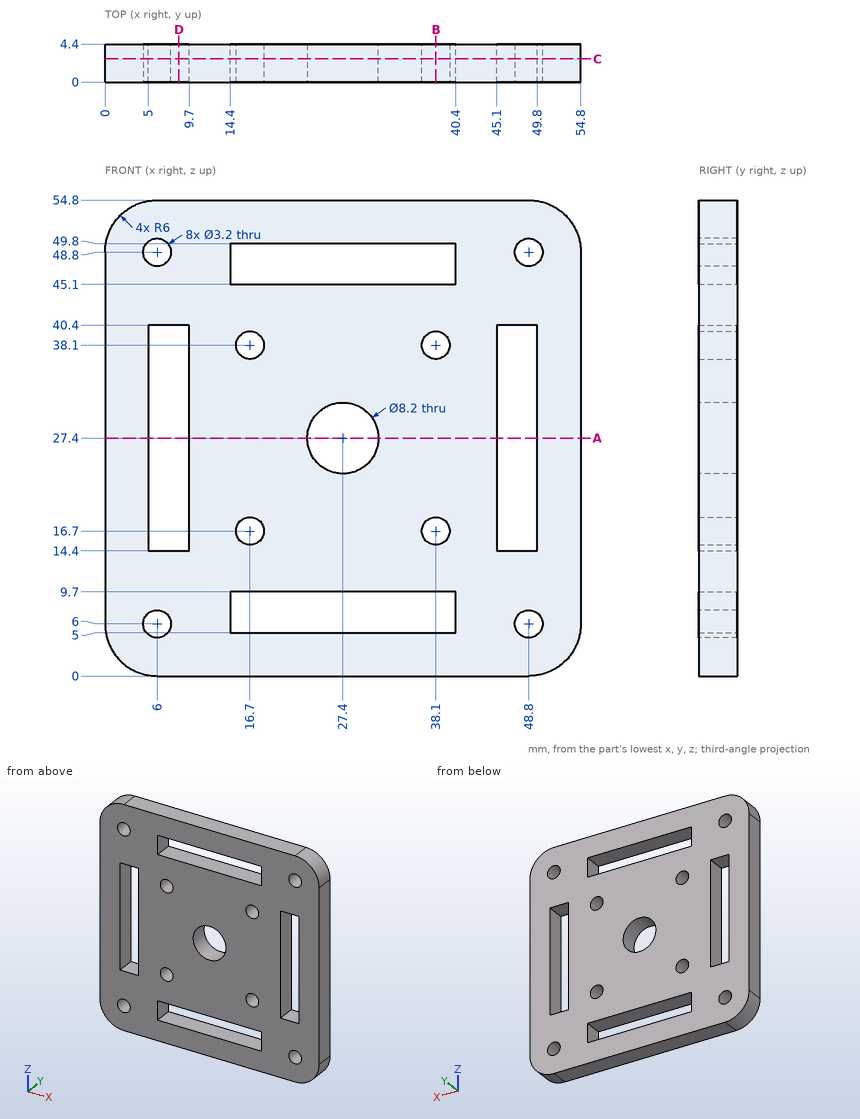
Answer from the drawing. Dimensions are ordinates in mm from the lowest x, y and z of the part. Give positions to 0.01 mm unless a question says otherwise; leave off trailing zeros. Order: outer loops, then holes, each group sorted by start corner. A loop starts at its lowest first (then second) coordinate and runs counter-clockwise, first axis right, second up. Notation, with made-up numbers: (-23, 72) - (6, 72) arc R10 cw to (6, 87) - close; hole circle Ø4 at (-10.75, -10). An arc over 180 degrees is marked (long way). One line per item, written item: value. Start each with the question number.
1) Find the intervals of material crossed by L1, parallel to Z at x = 16.7, y = 3; L2, parallel to X at y = 0.55, z = 22; L3, parallel to Z at x = 48.8, y = 2.65, in increasing order.
2) Given pin 1 Ø1.5 at (x, z) = (46.5, 35.5) entering from -Y, flat-ended and moving along its own axis, determine where the tip first touches the part or whether it passes through.
3) A cutting plane is placed at B-B on x = 38.1. Give the vertices of the cut face in (y, z).
4) A cutting plane is placed at A-A on z = 27.4. Give the vertices of the cut face in (x, y), then the cut area to 3 significant figures.
5) A cutting plane is placed at C-C on y = 2.7. State how many separate pieces and enclosed holes the cut face has, then the cut area to 3 significant figures.
6) A cutting plane is placed at D-D on x = 8.5. Give the vertices of the cut face in (y, z).
Answer sheet:
1. L1: z = 0 to 5, 9.7 to 15.1, 18.3 to 36.5, 39.7 to 45.1, 49.8 to 54.8
1. L2: x = 0 to 5, 9.7 to 45.1, 49.8 to 54.8
1. L3: z = 0 to 4.4, 7.6 to 14.4, 40.4 to 47.2, 50.4 to 54.8
2. pin 1: passes through
3. outline: (0, 0) - (4.4, 0) - (4.4, 5) - (0, 5) - close; (0, 9.7) - (4.4, 9.7) - (4.4, 15.1) - (0, 15.1) - close; (0, 18.3) - (4.4, 18.3) - (4.4, 36.5) - (0, 36.5) - close; (0, 39.7) - (4.4, 39.7) - (4.4, 45.1) - (0, 45.1) - close; (0, 49.8) - (4.4, 49.8) - (4.4, 54.8) - (0, 54.8) - close
4. outline: (0, 0) - (5, 0) - (5, 4.4) - (0, 4.4) - close; (9.7, 0) - (23.3, 0) - (23.3, 4.4) - (9.7, 4.4) - close; (31.5, 0) - (45.1, 0) - (45.1, 4.4) - (31.5, 4.4) - close; (49.8, 0) - (54.8, 0) - (54.8, 4.4) - (49.8, 4.4) - close
4. area: 164 mm2
5. separate pieces: 1
5. enclosed holes: 13
5. area: 2,370 mm2
6. outline: (0, 0) - (4.4, 0) - (4.4, 14.4) - (0, 14.4) - close; (0, 40.4) - (4.4, 40.4) - (4.4, 54.8) - (0, 54.8) - close
